```python
from build123d import *

# Parameters (mm, degrees)
SKETCH1_W           = 25.4
SKETCH1_H           = 50.8
SKETCH1_R           = 1.4605
SKETCH1_W_2         = 3.175
SKETCH1_H_2         = 25.4
BOSS_EXTRUDE1_DEPTH = 3.175


with BuildPart() as part:
    # Sketch1 → Boss-Extrude1 (new body)
    with BuildSketch(Plane(origin=(0, 0, 0), x_dir=(1, 0, 0), z_dir=(0, 1, 0))):
        with Locations((12.7, 25.4)):
            Rectangle(SKETCH1_W, SKETCH1_H)
        with Locations(Location((12.7, 13.97, 0), (0, 0, 270))):
            Circle(SKETCH1_R, mode=Mode.SUBTRACT)
        with Locations((9.525, 33.02)):
            Rectangle(SKETCH1_W_2, SKETCH1_H_2, mode=Mode.SUBTRACT)
        with Locations((15.875, 33.02)):
            Rectangle(SKETCH1_W_2, SKETCH1_H_2, mode=Mode.SUBTRACT)
    extrude(amount=BOSS_EXTRUDE1_DEPTH)


solid = part.part
```
Design review of the part built by this model. Coordinates are the model's own, in mm. A direction names the side the tool comes from. Round coordinates to 2 decimals unless told otherwise and drop trailing zeros. Write each loop counter-clockwise with the first axis right and the second up, starting at its lowest first coordinate (ties: lowest second). Pieces come first, ordered by that corner, then holes. Notation, with made-up numbers: (-33.5, 56) -> (18.5, 56) arc R17 cw to (18.5, 66) -> close; hole circle Ø2 at (25.5, 73). An arc over 180 degrees is marked (long way). Answer in a Markdown table with one row per item.
Q1. Take a section at D-D, the plane y = 1.4. State the section outline as (x, z) points, then the cut area to 3 significant figures.
The answers:
| item | result |
|---|---|
| outline | (0, -50.8) -> (25.4, -50.8) -> (25.4, 0) -> (0, 0) -> close; hole (7.94, -45.72) -> (11.11, -45.72) -> (11.11, -20.32) -> (7.94, -20.32) -> close; hole circle Ø2.92 at (12.7, -13.97); hole (14.29, -45.72) -> (17.46, -45.72) -> (17.46, -20.32) -> (14.29, -20.32) -> close |
| area | 1,120 mm² |
Q2. Take a section at C-C, the plane z = -13.97. State the section outline as (x, y) points (1 decimal), then the cut area to 3 significant figures.
The answers:
| item | result |
|---|---|
| outline | (0, 0) -> (11.2, 0) -> (11.2, 3.2) -> (0, 3.2) -> close; (14.2, 0) -> (25.4, 0) -> (25.4, 3.2) -> (14.2, 3.2) -> close |
| area | 71.4 mm² |
Q3. Take a section at B-B, the plane x = 12.7. State the section outline as (y, z) points (1 decimal), then the cut area to 3 significant figures.
The answers:
| item | result |
|---|---|
| outline | (0, -50.8) -> (3.2, -50.8) -> (3.2, -15.4) -> (0, -15.4) -> close; (0, -12.5) -> (3.2, -12.5) -> (3.2, 0) -> (0, 0) -> close |
| area | 152 mm² |
Q4. Clearance check with a flat-ended pin moving along its axis: pin 1 Ø12 at (x, z) = (19.5, -16) entering from -Y. State where the tip first meets the part, or that it passes through.
The answers:
| item | result |
|---|---|
| pin 1 | y = 0 |
Q5. To check wall thickness, follow L1, parallel to X at y = 1.95, z = -21.5; L2, parallel to X at y = 2.45, z = -13.97; L3, parallel to Z at x = 10.25, y = 1.85. State the ranges of each line that lie inside material, in increasing order. Write a range as [from, to].
The answers:
| item | result |
|---|---|
| L1 | [0, 7.94], [11.11, 14.29], [17.46, 25.4] |
| L2 | [0, 11.24], [14.16, 25.4] |
| L3 | [-50.8, -45.72], [-20.32, 0] |
Q6. For faces 1 (the face through (7.938, 2, -33)), 2 (the face through (25.4, 2, -25)), list the 3-axis set-ups (+Z, -Z, +X, -X, +Y, -Y) from which the entire face can be reached by the end or side of a thin tool; tool diameter is ignored.
The answers:
| item | result |
|---|---|
| face 1 | +Y, -Y |
| face 2 | +Z, -Z, +X, +Y, -Y |
Q7. Draft analysis for pull direction Z (two halves, no side actions). For faces 3 (the face through (16, 2, -45.72)), 4 (the face through (13, 3.175, -26)), 5 (the face through (11.274, 1.565, -14.287)), 6 (the face through (13, 2, -50.8)), state which applies: +Z half, -Z half, draft (parallel to the pull), parting line (faces both ways), or undercut.
The answers:
| item | result |
|---|---|
| face 3 | undercut |
| face 4 | draft |
| face 5 | undercut |
| face 6 | -Z half |
Q8. Take a section at A-A, the plane z = -21.5. State the section outline as (x, y) points (1 decimal).
The answers:
| item | result |
|---|---|
| outline | (0, 0) -> (7.9, 0) -> (7.9, 3.2) -> (0, 3.2) -> close; (11.1, 0) -> (14.3, 0) -> (14.3, 3.2) -> (11.1, 3.2) -> close; (17.5, 0) -> (25.4, 0) -> (25.4, 3.2) -> (17.5, 3.2) -> close |
